Verification items for this drawing (mm, ordinates from the low corner). A direction names the side the tool comes from. Coordinates: 2 decimals unless noted, no trailing zeros. Order: outer loops, then holes, each group sorted by start corner. A loop starts at its lowest first (then second) coordinate and runs counter-clockwise, first axis right, second up. Notation, with made-up numbers: M 85.25,6.25 L 102.25,6.25 A17 cw 102.25,15.25 Z; hole C 47,57.5 d4. An arc over 180 degrees is marked long. Answer as a JSON object with one key per item and string values. Group by question number.
(1) Mould release check, pull along X, two halves, no side actions. Record for the marked faces 1, 2, 3 and 4: released by +X, released by -X, zero draft, split by the parting line, or undercut.
(2) Gauge pin test, flat ends, axial feed: pin 1 Ø1.3 at (x, z) = (8, 0.5) entering from +Y; pin 2 Ø1.2 at (x, z) = (2.5, 8.5) entering from +Y; pin 3 Ø2 at (x, y) = (16.5, 3.5) entering from -Z. Record the tip position at first contact, or that the pin passes through.
(3) Access from +Z, -Z, +X, -X, +Y, -Y to the whole of each face (thin tool, end or side, straight path). Record for the marked faces 5 and 6.
(4) Cross-section at D-D (x = 14.5). Enter the section's corners in (y, z), plus the area to 3 significant figures.
(5) Cross-section at C-C (y = 1.8). Enter the section's corners in (x, z).
(6) Cross-section at B-B (z = 10.5). Enter the section's corners in (x, y).
(7) Cross-section at A-A (y = 4.55). Enter the section's corners in (x, z).
(8) Material ranges on line 1 (Z direction, x = 7, y = 3.75); line 2 (Z direction, x = 12.5, y = 3.4), recorded low to high.
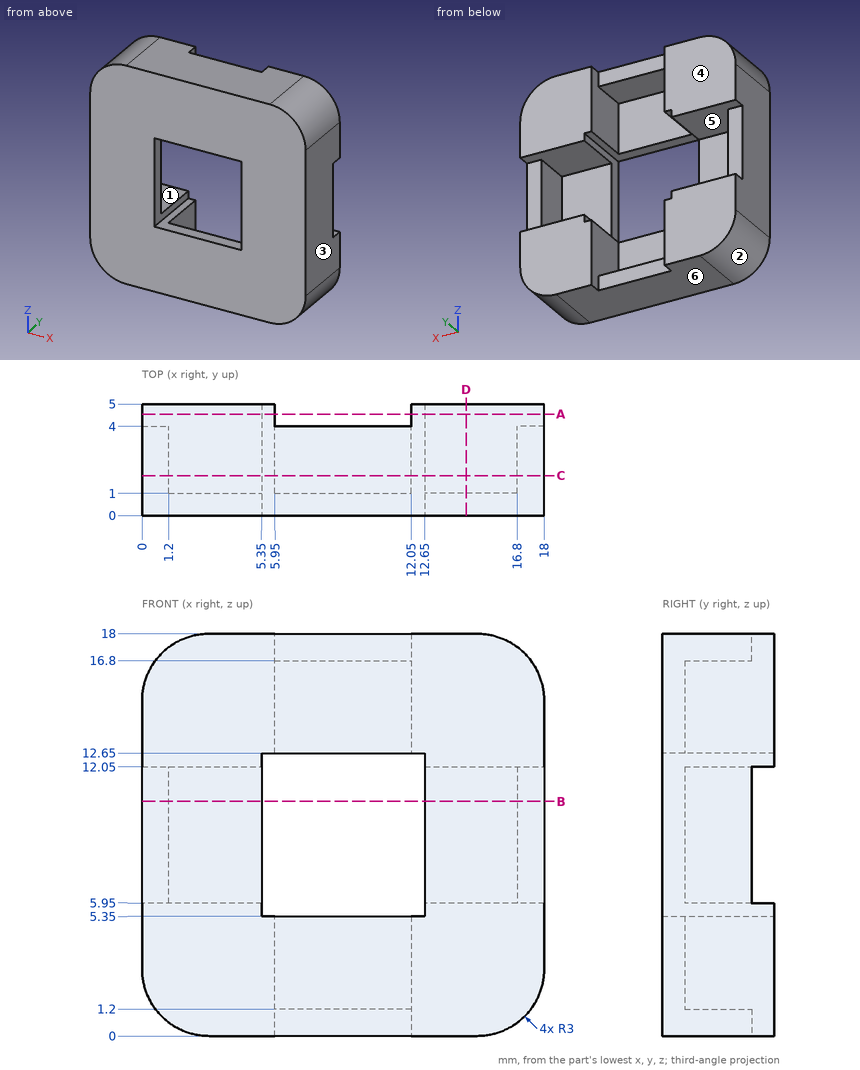
Taken from the geometry:
{
 "1": {"face 1": "undercut", "face 2": "released by -X", "face 3": "released by +X", "face 4": "zero draft"},
 "2": {"pin 1": "stops at y = 4", "pin 2": "stops at y = 1", "pin 3": "stops at z = 0.04"},
 "3": {"face 5": "+Y", "face 6": "-Z, +X, -X, +Y, -Y"},
 "4": {"outline": "M 0,0 L 5,0 L 5,5.95 L 1,5.95 L 1,12.05 L 5,12.05 L 5,18 L 0,18 Z", "area": "65.6 mm²"},
 "5": {"outline": "M 0,3 A3 ccw 3,0 L 15,0 A3 ccw 18,3 L 18,15 A3 ccw 15,18 L 3,18 A3 ccw 0,15 Z; hole M 1.2,5.95 L 5.35,5.95 L 5.35,5.35 L 5.95,5.35 L 5.95,1.2 L 12.05,1.2 L 12.05,5.35 L 12.65,5.35 L 12.65,5.95 L 16.8,5.95 L 16.8,12.05 L 12.65,12.05 L 12.65,12.65 L 12.05,12.65 L 12.05,16.8 L 5.95,16.8 L 5.95,12.65 L 5.35,12.65 L 5.35,12.05 L 1.2,12.05 Z"},
 "6": {"outline": "M 0,0 L 5.35,0 L 5.35,1 L 1.2,1 L 1.2,4 L 0,4 Z; M 12.65,0 L 18,0 L 18,4 L 16.8,4 L 16.8,1 L 12.65,1 Z"},
 "7": {"outline": "M 0,3 A3 ccw 3,0 L 5.95,0 L 5.95,5.35 L 5.35,5.35 L 5.35,5.95 L 0,5.95 Z; M 0,12.05 L 5.35,12.05 L 5.35,12.65 L 5.95,12.65 L 5.95,18 L 3,18 A3 ccw 0,15 Z; M 12.05,0 L 15,0 A3 ccw 18,3 L 18,5.95 L 12.65,5.95 L 12.65,5.35 L 12.05,5.35 Z; M 12.05,12.65 L 12.65,12.65 L 12.65,12.05 L 18,12.05 L 18,15 A3 ccw 15,18 L 12.05,18 Z"},
 "8": {"line 1": "z = 0 to 1.2, 16.8 to 18", "line 2": "z = 0 to 5.35, 12.65 to 18"}
}
